Check sheet for the drawn part. Datum: minimum x, y, z corner. Units: mm. A direction names the side the tool comes from. Give positions to 0.01 mm unless a question says otherwise; leave off trailing zeros. Order: outer loops, then holes, each group sorted by start corner. A loop starts at its lowest first (then second) coordinate and runs counter-clockwise, first axis right, second up. Notation, with made-up numbers: (-0.75, 20) - (48.25, 20) arc R15 cw to (48.25, 32) - close; hole circle Ø3 at (49.5, -38). An arc over 180 degrees is marked (long way). Answer as a JSON object with one key per item and string values. Group by question number.
(1) Thickness scan on line 1 (Z direction, x = 3.75, y = 5.75); line 2 (Z direction, x = 66.25, y = 8.5); line 3 (X direction, y = 12.25, z = 22). Record the ranges inside material, lowest first.
(2) Section check D-D (y = 3.25). Record the boundary of the cut face in (x, z).
(3) Section check C-C (z = 32.5). Record the boundary of the cut face in (x, y).
(4) Section check A-A (x = 66.25). Record the boundary of the cut face in (y, z).
(5) Depth check by flat-ended pin: pin 1 Ø6 at (x, z) = (52, 33.5) entering from +Y; pin 2 Ø5.5 at (x, z) = (37, 30) entering from +Y; pin 3 Ø4 at (y, z) = (7, 30) entering from +X. Enter the tip coordinate at first touch or a pass-through.
(6) Section check B-B (y = 7.25). Record the boundary of the cut face in (x, z).
(7) Mould release check, pull along Z, two halves, no side actions. Record for the marked faces 4, 5 and 6: +Z half, -Z half, draft (parallel to the pull), parting line (faces both ways), or undercut.
(8) Access from +Z, -Z, +X, -X, +Y, -Y to the whole of each face (thin tool, end or side, straight path). Record for the marked faces 1, 2 and 3.
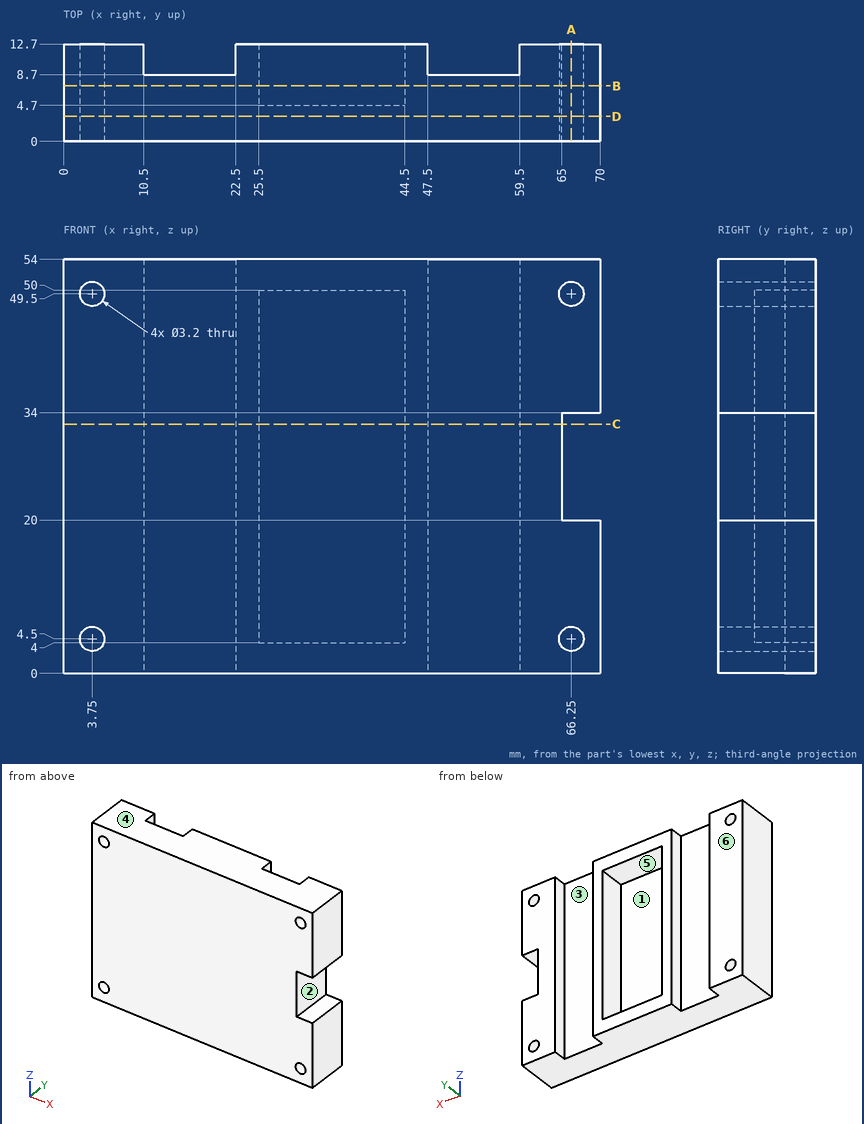
Solutions:
{
 "1": {"line 1": "z = 0 to 2.9, 6.1 to 47.9, 51.1 to 54", "line 2": "z = 0 to 2.9, 6.1 to 20, 34 to 47.9, 51.1 to 54", "line 3": "x = 0 to 10.5, 22.5 to 25.5, 44.5 to 47.5, 59.5 to 65"},
 "2": {"outline": "(0, 0) - (70, 0) - (70, 20) - (65, 20) - (65, 34) - (70, 34) - (70, 54) - (0, 54) - close; hole circle Ø3.2 at (3.75, 4.5); hole circle Ø3.2 at (3.75, 49.5); hole circle Ø3.2 at (66.25, 4.5); hole circle Ø3.2 at (66.25, 49.5)"},
 "3": {"outline": "(0, 0) - (65, 0) - (65, 12.7) - (59.5, 12.7) - (59.5, 8.7) - (47.5, 8.7) - (47.5, 12.7) - (44.5, 12.7) - (44.5, 4.7) - (25.5, 4.7) - (25.5, 12.7) - (22.5, 12.7) - (22.5, 8.7) - (10.5, 8.7) - (10.5, 12.7) - (0, 12.7) - close"},
 "4": {"outline": "(0, 0) - (12.7, 0) - (12.7, 2.9) - (0, 2.9) - close; (0, 6.1) - (12.7, 6.1) - (12.7, 20) - (0, 20) - close; (0, 34) - (12.7, 34) - (12.7, 47.9) - (0, 47.9) - close; (0, 51.1) - (12.7, 51.1) - (12.7, 54) - (0, 54) - close"},
 "5": {"pin 1": "stops at y = 8.7", "pin 2": "stops at y = 4.7", "pin 3": "stops at x = 65"},
 "6": {"outline": "(0, 0) - (70, 0) - (70, 20) - (65, 20) - (65, 34) - (70, 34) - (70, 54) - (0, 54) - close; hole circle Ø3.2 at (3.75, 4.5); hole circle Ø3.2 at (3.75, 49.5); hole (25.5, 4) - (44.5, 4) - (44.5, 50) - (25.5, 50) - close; hole circle Ø3.2 at (66.25, 4.5); hole circle Ø3.2 at (66.25, 49.5)"},
 "7": {"face 4": "+Z half", "face 5": "undercut", "face 6": "draft"},
 "8": {"face 1": "+Y", "face 2": "+X, +Y, -Y", "face 3": "+Z, -Z, +Y"}
}
